Part model, mm, in its own coordinate system. A direction names the side the tool comes from. Round coordinates to 2 decimals unless told otherwise and drop trailing zeros. Loops run counter-clockwise (first coordinate to the right, second up) from the corner with the lowest first, then second, coordinate; pieces in that order, holes last.
(1) Cut at B-B on x = -1. List the corners of the cut face in (y, z).
(2) Flat gauge pins, fed straight in: pin 1 (4 mm diameter, centred on x = 11.5, z = -4.5, fed in from +Y); pin 2 (4 mm diameter, centred on y = 10, z = 1, fed in from -X); pin 3 (4 mm diameter, centred on x = 0, y = -16, fed in from -Z); pin 4 (1.8 mm diameter, centred on x = 0, y = 16, fed in from +Z). Where does each tip first touch, or does it go through?
(3) Probe probe 1 along X at (y, z) = (-10, -0.25); probe 2 along Y at (x, z) = (0, 1.45); probe 3 along Y at (x, z) = (9, -4.5). List the from-to ranges inside material, lowest first.
(4) Cut at A-A on z = 1. List the corners of the cut face in (x, y) (3 decimals), then the cut area to 3 significant figures.
(5) Mould opens along Y. For faces 1 (the face through (7.879, -18.863, 0.986)), 2 (the face through (8.75, -9.95, 0.99)), 3 (the face through (-2, 18, 1)), 4 (the face through (4.31, -0.06, 0.99)) say: +Y half, -Y half, draft (parallel to the pull), parting line (faces both ways), or undercut.
(6) Cut at D-D on y = 5.5. List the corners of the cut face in (x, z), then the cut area to 3 significant figures.
(7) Cut at C-C on x = 2.25. List the corners of the cut face in (y, z).
(8) Tool access for faces 5 (the face through (7.904, 18.855, 0.986)), 6 (the face through (-2.6, 14.41, 0.99)): list every direction of +Z, -Z, +X, -X, +Y, -Y with a clear straight run to the whole face (end or side of a thin tool).
from build123d import *

# Parameters (mm, degrees)
F0_R     = 1.5
F0_R_2   = 2.6
F0_R_3   = 1.25
F1_DEPTH = 2


with BuildPart() as f1:
    # F0 (on Top) → F1 (new body)
    with BuildSketch(Plane.XY):
        with BuildLine():
            ThreePointArc((13.733325, -14.896663), (14.66458, -13.826485), (15, -12.448075))
            Line((15, -12.448075), (15, -2.025536))
            ThreePointArc((15, -2.025536), (13.859575, 0), (15, 2.025536))
            Line((15, 2.025536), (15, 12.448075))
            ThreePointArc((15, 12.448075), (14.66458, 13.826485), (13.733325, 14.896663))
            Line((13.733325, 14.896663), (8.715685, 18.448588))
            ThreePointArc((8.715685, 18.448588), (7.89182, 18.858825), (6.98236, 19))
            Line((6.98236, 19), (0.238068, 19))
            ThreePointArc((0.238068, 19), (-1.866179, 18.138258), (-2.761547, 16.048099))
            Line((-2.761547, 16.048099), (-2.774231, 15.257063))
            ThreePointArc((-2.774231, 15.257063), (-2.594506, 14.395821), (-2.062591, 13.695032))
            ThreePointArc((-2.062591, 13.695032), (4.30745, -0.287028), (-2.507604, -14.057665))
            ThreePointArc((-2.507604, -14.057665), (-3.061715, -14.741039), (-3.26896, -15.596076))
            Line((-3.26896, -15.596076), (-3.274666, -15.951901))
            ThreePointArc((-3.274666, -15.951901), (-2.41331, -18.104246), (-0.275051, -19))
            Line((-0.275051, -19), (6.98236, -19))
            ThreePointArc((6.98236, -19), (7.89182, -18.858825), (8.715685, -18.448588))
            Line((8.715685, -18.448588), (13.733325, -14.896663))
        make_face()
        with Locations((0, -16)):
            Circle(F0_R, mode=Mode.SUBTRACT)
        with Locations((10, -10)):
            Circle(F0_R_2, mode=Mode.SUBTRACT)
        with Locations((0, 16)):
            Circle(F0_R, mode=Mode.SUBTRACT)
        with Locations((10, 10)):
            Circle(F0_R_2, mode=Mode.SUBTRACT)
        with Locations((10, -10)):
            Circle(F0_R_2)
        with Locations((10, -10)):
            Circle(F0_R_3, mode=Mode.SUBTRACT)
        with Locations((10, 10)):
            Circle(F0_R_2)
        with Locations((10, 10)):
            Circle(F0_R_3, mode=Mode.SUBTRACT)
    extrude(amount=F1_DEPTH)

    # F4: sweep along a path in F3
    with BuildLine(Plane.YZ.offset(10)) as f4_path:
        Line((-7.331403, 0), (-9.867113, -5.437847))
    # F0 (on Top) → F4 (sweep)
    with BuildSketch(Plane.XY):
        with Locations((10, -10)):
            Circle(F0_R_2)
        with Locations((10, -10)):
            Circle(F0_R_3, mode=Mode.SUBTRACT)
    sweep(path=f4_path.line)

    # F5: sweep along a path in F3
    with BuildLine(Plane.YZ.offset(10)) as f5_path:
        Line((7.409177, 0), (9.944887, -5.437847))
    # F0 (on Top) → F5 (sweep)
    with BuildSketch(Plane.XY):
        with Locations((10, 10)):
            Circle(F0_R_2)
        with Locations((10, 10)):
            Circle(F0_R_3, mode=Mode.SUBTRACT)
    sweep(path=f5_path.line)


solid = f1.part
Final values:
1. outline: (-18.91, 0) - (-17.12, 0) - (-17.12, 2) - (-18.91, 2) - close; (-14.88, 0) - (-12.72, 0) - (-12.72, 2) - (-14.88, 2) - close; (12.72, 0) - (14.88, 0) - (14.88, 2) - (12.72, 2) - close; (17.12, 0) - (18.73, 0) - (18.73, 2) - (17.12, 2) - close
2. pin 1: stops at y = 15.14
2. pin 2: stops at x = -0.31
2. pin 3: stops at z = 0
2. pin 4: passes through
3. probe 1: x = 7.4 to 8.76, 11.24 to 12.6
3. probe 2: y = -19 to -17.5, -14.5 to -11.65, 11.65 to 14.5, 17.5 to 18.99
3. probe 3: y = -14.5 to -12.85, -11.35 to -9.7, 9.7 to 11.35, 12.85 to 14.5
4. outline: (-3.275, -15.952) arc R3 ccw to (-0.275, -19) - (6.982, -19) arc R3 ccw to (8.716, -18.449) - (13.733, -14.897) arc R3 ccw to (15, -12.448) - (15, -2.026) arc R2.369 cw to (15, 2.026) - (15, 12.448) arc R3 ccw to (13.733, 14.897) - (8.716, 18.449) arc R3 ccw to (6.982, 19) - (0.238, 19) arc R3 ccw to (-2.762, 16.048) - (-2.774, 15.257) arc R2 ccw to (-2.063, 13.695) arc R17.902 cw to (-2.508, -14.058) arc R2 ccw to (-3.269, -15.596) - close; hole circle Ø3 at (0, -16); hole circle Ø3 at (0, 16); hole circle Ø2.5 at (10, -10); hole circle Ø2.5 at (10, 10)
4. area: 469 mm2
5. face 1: -Y half
5. face 2: undercut
5. face 3: +Y half
5. face 4: undercut
6. outline: (3.44, 0) - (15, 0) - (15, 2) - (3.44, 2) - close
6. area: 23.1 mm2
7. outline: (-19, 0) - (-8.34, 0) - (-8.34, 2) - (-19, 2) - close; (8.34, 0) - (19, 0) - (19, 2) - (8.34, 2) - close
8. face 5: +Z, -Z, +X, +Y
8. face 6: +Z, -Z, -X
